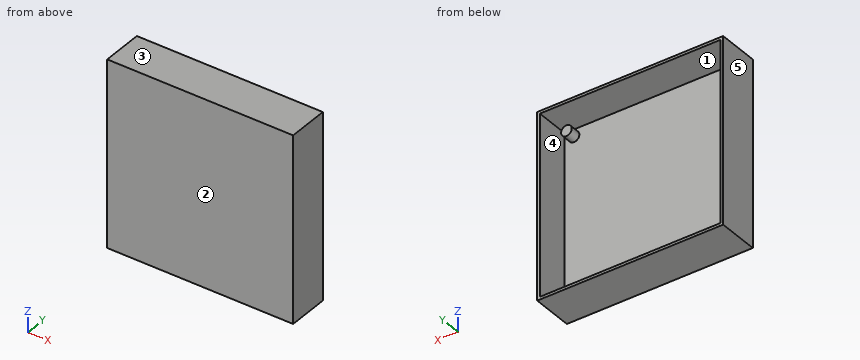
Solid Edge part; units mm, degrees
sketch "Sketch1" plane through (0, 0, 0) normal (0, -1, 0) x (1, 0, 0)
  line L0 (-35, -35) -> (35, -35)
  line L1 (35, -35) -> (35, 35)
  line L2 (35, 35) -> (-35, 35)
  line L3 (-35, 35) -> (-35, -35)
  dimension "D1" = 35
  dimension "D2" = 35
extrude "Protrusion1" add sketch "Sketch1" against normal blind 15.5
sketch "Sketch2" plane through (0, 15.5, 0) normal (0, 1, 0) x (0, 0, -1)
  line L0 (-34, -34) -> (34, -34)
  line L1 (34, -34) -> (34, 34)
  line L2 (34, 34) -> (-34, 34)
  line L3 (-34, 34) -> (-34, -34)
  dimension "D1" = 34
  dimension "D2" = 34
extrude "Enlèvement_matière_1" cut sketch "Sketch2" against normal blind 13
sketch "Sketch3" plane through (0, 2.5, 0) normal (0, 1, 0) x (0, 0, -1)
  circle A0 centre (-31.27, -30.485) radius 2
  circle A1 centre (-31.27, 30.485) radius 2
  dimension "D1" = 31.27
  dimension "D2" = 31.27
extrude "Ajout_matière_2" add sketch "Sketch3" along normal blind 4
Build history of the part. All positions in model axes, mm. Face numbers are marked on the shaded views. A direction names the side the tool comes from. Round coordinates to 2 decimals unless told otherwise and drop trailing zeros. Loops run counter-clockwise (first coordinate to the right, second up) from the corner with the lowest first, then second, coordinate; pieces in that order, holes last.
Item 1: Pin check, flat tips, straight feed: P1, Ø8, axis at x = 10.5, z = -13.5, coming from the +Y side; P2, Ø2, axis at x = 20.5, z = 28, coming from the -Y side; P3, Ø3, axis at x = 30, z = 31, coming from the +Y side. Stop position of each tip, or through.
Item 2: Saw through at B-B (z = 31.27). List the corners of the cut face in (x, y) (3 decimals).
Item 3: Drill centre lines: line 1 along Z through (x, y) = (25.5, 3); line 2 along Y through (x, z) = (29, -26.5). Where is each one in solid material? Low to high.
Item 4: Saw through at C-C (x = 15.5). List the corners of the cut face in (y, z), then the cut area to 3 significant figures.
Item 5: Saw through at A-A (y = 11.25). List the corners of the cut face in (x, z).
Item 6: Two-plate mould, pull along Z, no slides. Class the marked faces 3, 4 and 5: released by +Z, released by -Z, zero draft, split by the parting line, or undercut.
Item 7: Saw through at D-D (z = 12.5). List the corners of the cut face in (x, y), then the cut area to 3 significant figures.
Item 8: Which spindle directions (+Z, -Z, +X, -X, +Y, -Y) get a long thin tool onto all of the face, cutting with end or side? Do the marked faces 1 and 2. Say none if no direction does.
Worked answers:
1. P1: stops at y = 2.5
1. P2: stops at y = 0
1. P3: stops at y = 6.5
2. outline: (-35, 0) - (35, 0) - (35, 15.5) - (34, 15.5) - (34, 2.5) - (32.485, 2.5) - (32.485, 6.5) - (28.485, 6.5) - (28.485, 2.5) - (-28.485, 2.5) - (-28.485, 6.5) - (-32.485, 6.5) - (-32.485, 2.5) - (-34, 2.5) - (-34, 15.5) - (-35, 15.5) - close
3. line 1: z = -35 to -34, 34 to 35
3. line 2: y = 0 to 2.5
4. outline: (0, -35) - (15.5, -35) - (15.5, -34) - (2.5, -34) - (2.5, 34) - (15.5, 34) - (15.5, 35) - (0, 35) - close
4. area: 201 mm2
5. outline: (-35, -35) - (35, -35) - (35, 35) - (-35, 35) - close; hole (-34, -34) - (34, -34) - (34, 34) - (-34, 34) - close
6. face 3: released by +Z
6. face 4: undercut
6. face 5: zero draft
7. outline: (-35, 0) - (35, 0) - (35, 15.5) - (34, 15.5) - (34, 2.5) - (-34, 2.5) - (-34, 15.5) - (-35, 15.5) - close
7. area: 201 mm2
8. face 1: +Y
8. face 2: +Z, -Z, +X, -X, -Y
